```python
from build123d import *

# Parameters (mm, degrees)
SKETCH2_R           = 27.469
BOSS_EXTRUDE1_DEPTH = 4
SKETCH3_R           = 2
CUT_EXTRUDE1_DEPTH  = 5


with BuildPart() as part:
    # Sketch2 → Boss-Extrude1 (new body)
    with BuildSketch(Plane(origin=(0, 0, 0), x_dir=(1, 0, 0), z_dir=(0, 1, 0))):
        Circle(SKETCH2_R)
    extrude(amount=BOSS_EXTRUDE1_DEPTH)

    # Sketch3 → Cut-Extrude1 (cut, through all)
    with BuildSketch(Plane(origin=(0, 4, 0), x_dir=(1, 0, 0), z_dir=(0, 1, 0))):
        with Locations((-23.971, 0)):
            Circle(SKETCH3_R)
        with Locations((0, 23.971)):
            Circle(SKETCH3_R)
        with Locations((23.971, 0)):
            Circle(SKETCH3_R)
        with Locations((0, -23.971)):
            Circle(SKETCH3_R)
    extrude(amount=-CUT_EXTRUDE1_DEPTH, mode=Mode.SUBTRACT)


solid = part.part
```
Geometry: final body of the model. Coordinates: model frame, mm. Round coordinates to 2 decimals unless told otherwise and drop trailing zeros. Loops run counter-clockwise (first coordinate to the right, second up) from the corner with the lowest first, then second, coordinate; pieces in that order, holes last. Notation, with made-up numbers: (51, 52.25) -> (56, 52.25) arc R31 cw to (56, 84.25) -> close; hole circle Ø1 at (4, -17). An arc over 180 degrees is marked (long way). Use one line per item in the form item = value. Start each with the question number.
1) Line query: L1, parallel to Z at x = 0, y = 1.25; L2, parallel to Z at x = -1.5, y = 1.75. Output: solid intervals per line, ascending.
2) First-contact query: P1, Ø6.5, axis at x = -23.971, z = 0, coming from the -Y side; P2, Ø1.5, axis at x = 6.5, y = 3.5, coming from the +Z side. Flat tips, straight axial feed; report the tip coordinate or a pass-through.
3) Section A-A on x = 0. Output: boundary loops of the cut face in (y, z).
4) Section D-D on z = 13. Output: boundary loops of the cut face in (x, y), then the cut area to 3 significant figures.
5) Draft query along X for faces 1 (the flat face through (0, 0, 0)), 2 (the cylindrical face through (12.675, 1.972, 24.37)), 3 (the cylindrical face through (-0.434, 2.028, -22.019)), 4 (the cylindrical face through (-25.97, 2.03, -0.09)). Return one class per face: released by +X, released by -X, zero draft, split by the parting line, or undercut.
6) Section C-C on y = 1.9. Output: boundary loops of the cut face in (x, z), then the cut area to 3 significant figures.
7) Section B-B on z = 0. Output: boundary loops of the cut face in (x, y).
Response:
q1.L1 = -27.47 to -25.97, -21.97 to 21.97, 25.97 to 27.47
q1.L2 = -27.43 to -25.29, -22.65 to 22.65, 25.29 to 27.43
q2.P1 = 0
q2.P2 = 26.86
q3.outline = (0, -27.47) -> (4, -27.47) -> (4, -25.97) -> (0, -25.97) -> close; (0, -21.97) -> (4, -21.97) -> (4, 21.97) -> (0, 21.97) -> close; (0, 25.97) -> (4, 25.97) -> (4, 27.47) -> (0, 27.47) -> close
q4.outline = (-24.2, 0) -> (24.2, 0) -> (24.2, 4) -> (-24.2, 4) -> close
q4.area = 194 mm^2
q5.face_1 = zero draft
q5.face_2 = split by the parting line
q5.face_3 = undercut
q5.face_4 = undercut
q6.outline = circle Ø54.94 at (0, 0); hole circle Ø4 at (-23.97, 0); hole circle Ø4 at (0, -23.97); hole circle Ø4 at (0, 23.97); hole circle Ø4 at (23.97, 0)
q6.area = 2,320 mm^2
q7.outline = (-27.47, 0) -> (-25.97, 0) -> (-25.97, 4) -> (-27.47, 4) -> close; (-21.97, 0) -> (21.97, 0) -> (21.97, 4) -> (-21.97, 4) -> close; (25.97, 0) -> (27.47, 0) -> (27.47, 4) -> (25.97, 4) -> close
